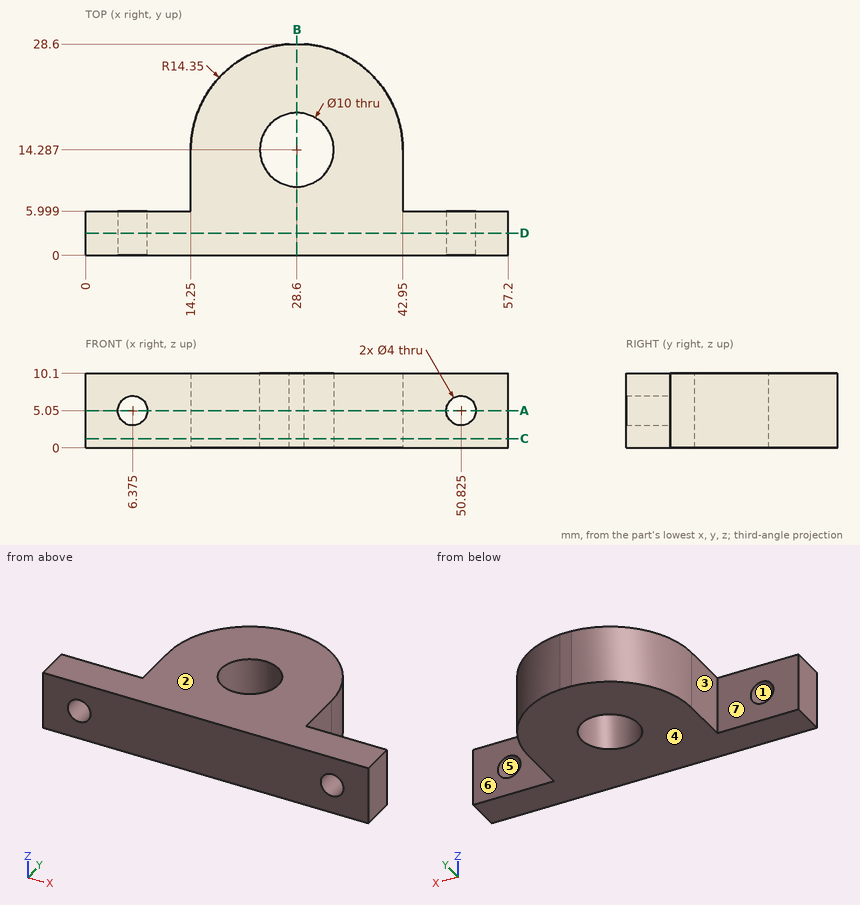
Study the drawing (mm; zero at the part's minimum x, y, z) and answer. A direction names the side the tool comes from. Round coordinates to 2 decimals unless told otherwise and drop trailing zeros. Loops run counter-clockwise (first coordinate to the right, second up) from the corner with the lowest first, then second, coordinate; pieces in that order, holes last.
Q1. Section C-C, the plane z = 1.25 is taken. Determine the outline of the cut face in (x, y).
Q2. Find the intervals of material crossed by line 1 (Y direction, x = 28.6, z = 8); line 2 (X direction, y = 4.75, z = 4.25); line 3 (Y direction, x = 4, z = 6.25), in increasing order.
Q3. Given pin 1 Ø4 at (y, z) = (15, 2) entering from -X; pin 2 Ø2 at (y, z) = (10.5, 4) entering from +X; pin 3 Ø12 at (x, y) = (23, 16.5) entering from -Z; pin 4 Ø3 at (x, z) = (33, 8.5) entering from +Y, each flat-ended and moving along its own axis, determine where each tip first touches the part or whether it passes through.
Q4. For a pull along Z with two mould halves and no side action, classify the marked faces 1, 2, 3 and 4 as released by +Z, released by -Z, zero draft, split by the parting line, or undercut.
Q5. Section D-D, the plane y = 3 is taken. Determine the outline of the cut face in (x, z) (3 decimals), then the cut area to 3 significant figures.
Q6. Section A-A, the plane z = 5.05 is taken. Determine the outline of the cut face in (x, y) (3 decimals), then the cut area to 3 significant figures.
Q7. Which of the six approach directions +Z, -Z, +X, -X, +Y, -Y give full straight-line access (tool end or side, diameter ignored) to the marked faces 5, 6 and 7?
Q8. Section B-B, the plane x = 28.6 is taken. Determine the outline of the cut face in (y, z), then the cut area to 3 significant figures.
Completed:
1. outline: (0, 0) - (57.2, 0) - (57.2, 6) - (42.95, 6) - (42.95, 14.29) arc R14.35 ccw to (29.63, 28.6) - (27.57, 28.6) arc R14.35 ccw to (14.25, 14.29) - (14.25, 6) - (0, 6) - close; hole circle Ø10 at (28.6, 14.29)
2. line 1: y = 0 to 9.29, 19.29 to 28.6
2. line 2: x = 0 to 4.54, 8.21 to 48.99, 52.66 to 57.2
2. line 3: y = 0 to 6
3. pin 1: stops at x = 14.25
3. pin 2: stops at x = 42.95
3. pin 3: stops at z = 0
3. pin 4: stops at y = 28.34
4. face 1: undercut
4. face 2: released by +Z
4. face 3: zero draft
4. face 4: released by -Z
5. outline: (0, 0) - (57.2, 0) - (57.2, 10.1) - (0, 10.1) - close; hole circle Ø4 at (6.375, 5.05); hole circle Ø4 at (50.825, 5.05)
5. area: 553 mm2
6. outline: (0, 0) - (4.375, 0) - (4.375, 5.999) - (0, 5.999) - close; (8.375, 0) - (48.825, 0) - (48.825, 5.999) - (42.95, 5.999) - (42.95, 14.287) arc R14.35 ccw to (29.63, 28.6) - (27.57, 28.6) arc R14.35 ccw to (14.25, 14.287) - (14.25, 5.999) - (8.375, 5.999) - close; (52.825, 0) - (57.2, 0) - (57.2, 5.999) - (52.825, 5.999) - close; hole circle Ø10 at (28.6, 14.287)
6. area: 778 mm2
7. face 5: +Y, -Y
7. face 6: +Z, -Z, +X, +Y
7. face 7: +Z, -Z, -X, +Y
8. outline: (0, 0) - (9.29, 0) - (9.29, 10.1) - (0, 10.1) - close; (19.29, 0) - (28.6, 0) - (28.6, 10.1) - (19.29, 10.1) - close
8. area: 188 mm2
